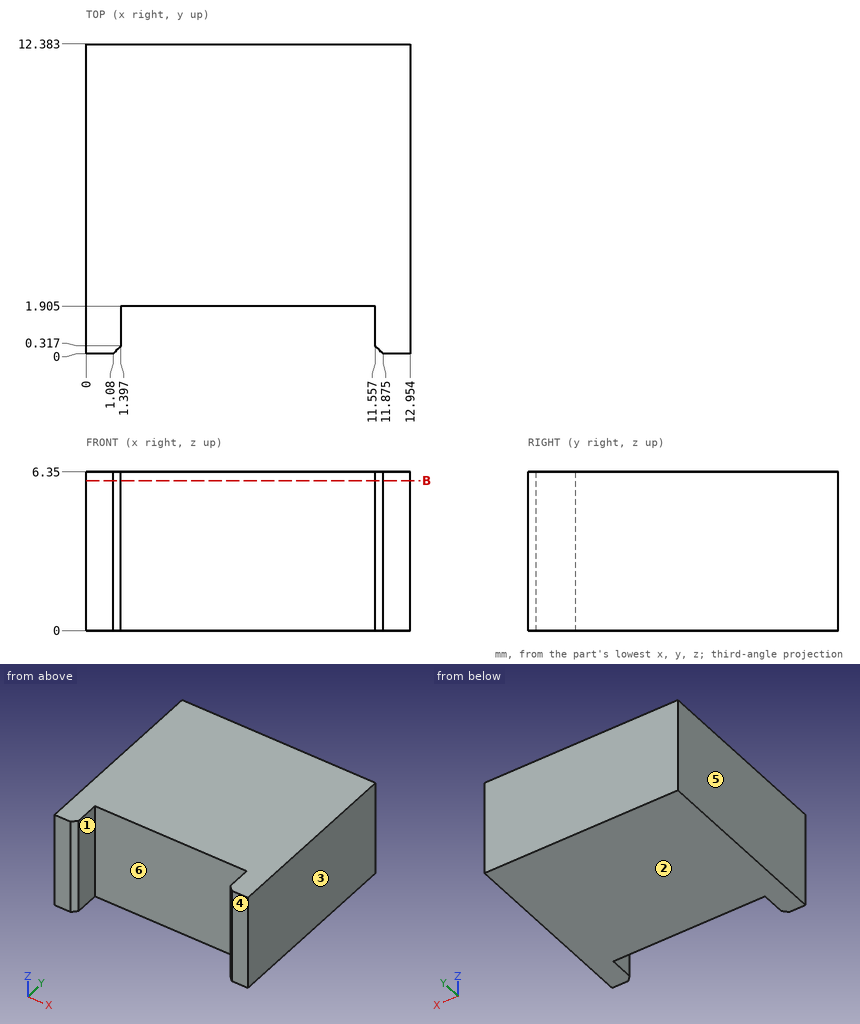
Part print with two shaded views. Sizes in mm from the minimum x, y, z corner. A direction names the side the tool comes from. Round coordinates to 2 decimals unless told otherwise and drop trailing zeros. Write each loop counter-clockwise with the first axis right and the second up, starting at its lowest first coordinate (ties: lowest second). Pieces come first, ordered by that corner, then holes. Notation, with made-up numbers: M -29.5,36 L 1.5,36 A12 cw 1.5,49 Z; hole C 0,88 d11. An arc over 180 degrees is marked long. Put each result on its own line as item: value. Start each with the question number.
1) Saw through at B-B, the plane z = 6. Write the cut outline in (x, y) (1 decimal), and give its area (3 significant figures).
2) Drill centre line: probe 1 along Y at (x, z) = (2, 3.75) (1 decimal). Where is it in solid material? Low to high. Write a range as [from, to].
3) Pull direction X, two halves, no side cores. Call the marked faces 3, 4, 5 and 6: pulls with the +X half, pulls with the -X half, needs draft (parallel to the pull), parting line crosses it, or undercut.
4) 3-axis set-ups, long thin cutter, end or side, ignore diameter. For the marked faces 1 and 2: which of +Z, -Z, +X, -X, +Y, -Y reach the whole face in a straight line?
Resolved:
1. outline: M 0,0 L 1.1,0 L 1.4,0.3 L 1.4,1.9 L 11.6,1.9 L 11.6,0.3 L 11.9,0 L 13,0 L 13,12.4 L 0,12.4 Z
1. area: 141 mm²
2. probe 1: [1.9, 12.4]
3. face 3: pulls with the +X half
3. face 4: needs draft
3. face 5: pulls with the -X half
3. face 6: undercut
4. face 1: +Z, -Z, -Y
4. face 2: -Z, +X, -X, +Y, -Y
